```python
from build123d import *

# Parameters (mm, degrees)
CROQUIS2_W              = 850
CROQUIS2_H              = 250
SALIENTE_EXTRUIR1_DEPTH = 150
CROQUIS3_R              = 75
CORTAR_EXTRUIR1_DEPTH   = 50
CROQUIS4_R              = 75
SALIENTE_EXTRUIR2_DEPTH = 50


with BuildPart() as part:
    # Croquis2 → Saliente-Extruir1 (new body)
    with BuildSketch(Plane.XY.offset(3.171613416)):
        with Locations((916.834843653, 1024.026997685)):
            Rectangle(CROQUIS2_W, CROQUIS2_H)
    extrude(amount=SALIENTE_EXTRUIR1_DEPTH)

    # Croquis3 → Cortar-Extruir1 (cut)
    with BuildSketch(Plane(origin=(0, 0, 3.171613416), x_dir=(-1, 0, 0), z_dir=(0, 0, -1))):
        with Locations((-616.834843653, 1024.026997685)):
            Circle(CROQUIS3_R)
    extrude(amount=-CORTAR_EXTRUIR1_DEPTH, mode=Mode.SUBTRACT)

    # Croquis4 → Saliente-Extruir2 (add)
    with BuildSketch(Plane.XY.offset(153.171613416)):
        with Locations((1216.834843653, 1024.026997685)):
            Circle(CROQUIS4_R)
    extrude(amount=SALIENTE_EXTRUIR2_DEPTH)


solid = part.part
```
Source: CAD feature listing. Evaluate the final solid. Frame: model axes, mm. A direction names the side the tool comes from. Round coordinates to 2 decimals unless told otherwise and drop trailing zeros. Loops run counter-clockwise (first coordinate to the right, second up) from the corner with the lowest first, then second, coordinate; pieces in that order, holes last.
1. Section query B-B on x = 1179. Output: boundary loops of the cut face in (y, z).
2. Section query D-D on z = 168. Output: boundary loops of the cut face in (x, y), and give its area (3 significant figures).
3. Section query C-C on y = 918.5. Output: boundary loops of the cut face in (x, z), and give its area (4 significant figures).
4. Access query for faces 1 (the flat face through (1216, 1025, 203.172)), 2 (the flat face through (618, 1025, 53.172)). Directions: +Z, -Z, +X, -X, +Y, -Y. A direction counts if a zero-diameter tool reaches every point of the face in a straight line with its end or side. Return the directions, or none.
5. Mould query, pull axis X, two halves, no side actions, for faces 3 (the flat face through (491.835, 1022, 77)), 4 (the cylindrical face through (1257.15, 1087.27, 177.82)), 5 (the flat face through (911, 1026, 153.172)), 6 (the cylindrical face through (672.11, 1074.72, 27.82)). Classes: released by +X, released by -X, zero draft, split by the parting line, or undercut.
6. Contact query for flat-ended pins moving along their axis: pin 1 (1 mm diameter, centred on x = 1247.5, y = 945.5, fed in from +Z); pin 2 (3 mm diameter, centred on x = 1176.5, z = 169.5, fed in from -Y). Output: stop coordinate, or through.
7. Section query A-A on z = 24.5. Output: boundary loops of the cut face in (x, y).
8. Ray query, L1, parallel to Z at x = 751.5, y = 1131; L2, parallel to X at y = 1040, z = 41; L3, parallel to X at y = 1007.5, z = 44.5. Return the intervals inside material, ascending.
Answers below:
1. outline: (899.03, 3.17) - (1149.03, 3.17) - (1149.03, 153.17) - (1088.78, 153.17) - (1088.78, 203.17) - (959.27, 203.17) - (959.27, 153.17) - (899.03, 153.17) - close
2. outline: circle Ø150 at (1216.83, 1024.03)
2. area: 17,700 mm2
3. outline: (491.83, 3.17) - (1341.83, 3.17) - (1341.83, 153.17) - (491.83, 153.17) - close
3. area: 127,500 mm2
4. face 1: +Z, +X, -X, +Y, -Y
4. face 2: -Z
5. face 3: released by -X
5. face 4: split by the parting line
5. face 5: zero draft
5. face 6: undercut
6. pin 1: stops at z = 153.17
6. pin 2: stops at y = 959.86
7. outline: (491.83, 899.03) - (1341.83, 899.03) - (1341.83, 1149.03) - (491.83, 1149.03) - close; hole circle Ø150 at (616.83, 1024.03)
8. L1: z = 3.17 to 153.17
8. L2: x = 491.83 to 543.56, 690.11 to 1341.83
8. L3: x = 491.83 to 543.68, 689.99 to 1341.83
